Geometry: final body of the model. Coordinates: model frame, mm. Face numbers are marked on the shaded views. A direction names the side the tool comes from. Round coordinates to 2 decimals unless told otherwise and drop trailing zeros. Write each loop counter-clockwise with the first axis right and the second up, starting at its lowest first coordinate (ties: lowest second). Pieces come first, ordered by that corner, then holes. Notation, with made-up numbers: (44.5, 29) -> (52.5, 29) arc R14 cw to (52.5, 40) -> close; hole circle Ø2 at (87, 31). An arc over 180 degrees is marked (long way). One line per item, written item: value. Start each with the question number.
from build123d import *

# Parameters (mm, degrees)
CUT_EXTRUDE1_DEPTH      = 68.23495628
CUT_EXTRUDE1_DEPTH_BACK = 68.23495628
SKETCH3_R               = 17.78
CUT_EXTRUDE2_DEPTH      = 51.816
CUT_EXTRUDE3_DEPTH      = 68.234956346
CUT_EXTRUDE3_DEPTH_BACK = 68.234956346
SKETCH4_R               = 6.35
CUT_EXTRUDE4_START      = 22.225
SKETCH5_W               = 22.352
SKETCH5_H               = 19.05
CUT_EXTRUDE4_DEPTH      = 3.048


with BuildPart() as part:
    # Sketch1 → Revolve1 (revolve)
    with BuildSketch(Plane.XY, mode=Mode.PRIVATE) as revolve1_sk:
        with BuildLine():
            Line((0, 0), (0, 58.166))
            ThreePointArc((0, 58.166), (6.387986381, 58.484288237), (12.712693656, 59.436))
            Line((12.712693656, 59.436), (22.225, 59.436))
            Line((22.225, 59.436), (22.225, 51.816))
            Line((22.225, 51.816), (19.685, 51.816))
            Line((19.685, 51.816), (19.685, 49.276))
            Line((19.685, 49.276), (22.225, 49.276))
            Line((22.225, 49.276), (22.225, 46.736))
            Line((22.225, 46.736), (19.685, 46.736))
            Line((19.685, 46.736), (19.685, 44.196))
            Line((19.685, 44.196), (22.225, 44.196))
            Line((22.225, 44.196), (22.225, 0))
            Line((22.225, 0), (0, 0))
        make_face()
    revolve(revolve1_sk.sketch.rotate(Axis((0, 59.436, 0), (0, 1, 0)), 90), axis=Axis((0, 59.436, 0), (0, 1, 0)))

    # Sketch2 → Cut-Extrude1 (cut, two sides: drawn at the far end of the back side and taken through both)
    with BuildSketch(Plane.XY.offset(-CUT_EXTRUDE1_DEPTH_BACK)):
        with BuildLine():
            Line((22.225, 0), (22.225, 7.62))
            Line((22.225, 7.62), (13.470533586, 7.62))
            ThreePointArc((13.470533586, 7.62), (11.673046061, 7.169336035), (10.300788381, 5.923957269))
            Line((10.300788381, 5.923957269), (6.35, 0))
            Line((6.35, 0), (22.225, 0))
        make_face()
        with BuildLine():
            Line((-22.225, 0), (-22.225, 7.62))
            Line((-22.225, 7.62), (-13.470533586, 7.62))
            ThreePointArc((-13.470533586, 7.62), (-11.673046061, 7.169336035), (-10.300788381, 5.923957269))
            Line((-10.300788381, 5.923957269), (-6.35, 0))
            Line((-6.35, 0), (-22.225, 0))
        make_face()
    extrude(amount=CUT_EXTRUDE1_DEPTH + CUT_EXTRUDE1_DEPTH_BACK, mode=Mode.SUBTRACT)

    # Sketch3 → Cut-Extrude2 (cut)
    with BuildSketch(Plane.XZ):
        with Locations(Location((0, 0, 0), (0, 0, 270))):
            Circle(SKETCH3_R)
    extrude(amount=-CUT_EXTRUDE2_DEPTH, mode=Mode.SUBTRACT)

    # Sketch4 → Cut-Extrude3 (cut, two sides: drawn at the far end of the back side and taken through both)
    with BuildSketch(Plane.XY.offset(-CUT_EXTRUDE3_DEPTH_BACK)):
        with Locations((0, 30.48)):
            Circle(SKETCH4_R)
    extrude(amount=CUT_EXTRUDE3_DEPTH + CUT_EXTRUDE3_DEPTH_BACK, mode=Mode.SUBTRACT)

    # Sketch5 → Cut-Extrude4 (cut)
    with BuildSketch(Plane.XY.offset(CUT_EXTRUDE4_START)):
        with Locations((0, 30.48)):
            Rectangle(SKETCH5_W, SKETCH5_H)
    extrude(amount=-CUT_EXTRUDE4_DEPTH, mode=Mode.SUBTRACT)


solid = part.part
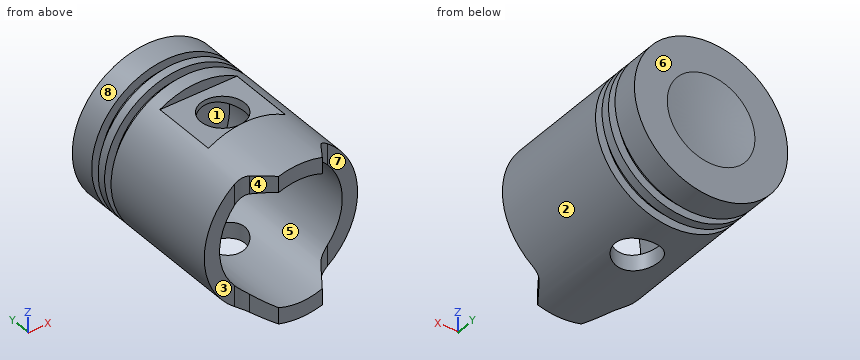
(1) Pin query (flat end, axial travel): pin 1 (5 mm diameter, centred on y = 18.5, z = -12.5, fed in from +X); pin 2 (13.5 mm diameter, centred on x = 10, z = 1.5, fed in from -Y); pin 3 (12 mm diameter, centred on x = 10.5, y = 8, fed in from -Z). Return the tip coordinate at first contact, or that it passes through.
(2) Section query A-A (y = 30.48). Output: boundary loops of the cut face in (x, z) (3 decimals).
(3) Section query B-B (z = 0). Output: boundary loops of the cut face in (x, y) (3 decimals).
(4) Pull-direction query (X, two-part tool) for the marked faces 1, 2, 3 and 4; classes: pulls with the +X half, pulls with the -X half, needs draft (parallel to the pull), parting line crosses it, or undercut.
(5) Line query: probe 1 along Y at (x, z) = (16, -12.5); probe 2 along X at (y, z) = (18, 0) (3 decimals); probe 3 along Y at (x, z) = (-11, 8). Output: solid intervals per line, ascending.
(6) Set-up query: the marked faces 5, 6, 7 and 8. Return all of +Z, -Z, +X, -X, +Y, -Y with unobstructed straight access to the full face (end or side cutting, diameter ignored); none if empty.
(7) Section query C-C (x = 0). Count the separate pieces of the cut face and the enclosed holes in it, and give its area (3 significant figures).
(8) Section query D-D (y = 19). Output: boundary loops of the cut face in (x, z) (3 decimals).
Results list:
1. pin 1: stops at x = 19.85
1. pin 2: stops at y = 51.82
1. pin 3: stops at z = -21.76
2. outline: (-11.176, 19.177) -> (-11.176, 19.211) arc R22.225 ccw to (-6.35, -21.299) -> (-6.35, -16.607) arc R17.78 cw to (-6.35, 16.607) -> (-6.35, 19.177) -> close; (6.35, -21.299) arc R22.225 ccw to (11.176, 19.211) -> (11.176, 19.177) -> (6.35, 19.177) -> (6.35, 16.607) arc R17.78 cw to (6.35, -16.607) -> close
3. outline: (-22.225, 7.62) -> (-17.78, 7.62) -> (-17.78, 51.816) -> (17.78, 51.816) -> (17.78, 7.62) -> (22.225, 7.62) -> (22.225, 44.196) -> (19.685, 44.196) -> (19.685, 46.736) -> (22.225, 46.736) -> (22.225, 49.276) -> (19.685, 49.276) -> (19.685, 51.816) -> (22.225, 51.816) -> (22.225, 59.436) -> (12.713, 59.436) arc R64.262 cw to (-12.713, 59.436) -> (-22.225, 59.436) -> (-22.225, 51.816) -> (-19.685, 51.816) -> (-19.685, 49.276) -> (-22.225, 49.276) -> (-22.225, 46.736) -> (-19.685, 46.736) -> (-19.685, 44.196) -> (-22.225, 44.196) -> close
4. face 1: undercut
4. face 2: parting line crosses it
4. face 3: needs draft
4. face 4: pulls with the -X half
5. probe 1: y = 7.62 to 44.2, 46.74 to 49.28, 51.82 to 59.44
5. probe 2: x = -22.225 to -17.78, 17.78 to 22.225
5. probe 3: y = 51.82 to 59.44
6. face 5: -Y
6. face 6: +Z, -Z, +X, -X, +Y
6. face 7: +Z, -Z, +X, -Y
6. face 8: +Y, -Y
7. separate pieces: 3
7. enclosed holes: 0
7. area: 620 mm^2
8. outline: circle Ø44.45 at (0, 0); hole circle Ø35.56 at (0, 0)
